```python
from build123d import *

# Parameters (mm, degrees)
PAD006_DEPTH    = 40
SKETCH009_W     = 14
SKETCH009_H     = 39
POCKET002_DEPTH = 5
SKETCH010_R     = 8.1
POCKET003_DEPTH = 5
FILLET001_R     = 3
FILLET002_R     = 2
FILLET003_R     = 4
CHAMFER_SIZE    = 2
CHAMFER001_SIZE = 2


with BuildPart() as part:
    # Sketch008 → Pad006 (new body, symmetric)
    with BuildSketch(Plane.YZ):
        Polygon((97.701339, 0), (115.394972, 0), (113.719903, 25.952241), (111.219903, 25.952241), (112.701339, 3), (97.701339, 3), align=None)
    extrude(amount=PAD006_DEPTH, both=True)

    # Sketch009 (on Face5 of Pad006) → Pocket002 (cut)
    with BuildSketch(Plane(origin=(0, 0, 3), x_dir=(0, -1, 0), z_dir=(0, 0, 1))):
        with Locations((-100.701339, 0)):
            Rectangle(SKETCH009_W, SKETCH009_H)
        with BuildLine():
            ThreePointArc((-103.101339, -36.625), (-101.401339, -38.325), (-99.701339, -36.625))
            Line((-99.701339, -36.625), (-99.701339, -33.225))
            ThreePointArc((-99.701339, -33.225), (-101.401339, -31.525), (-103.101339, -33.225))
            Line((-103.101339, -36.625), (-103.101339, -33.225))
        make_face()
        with BuildLine():
            ThreePointArc((-103.101339, 33.225), (-101.401339, 31.525), (-99.701339, 33.225))
            Line((-99.701339, 33.225), (-99.701339, 36.625))
            ThreePointArc((-99.701339, 36.625), (-101.401339, 38.325), (-103.101339, 36.625))
            Line((-103.101339, 33.225), (-103.101339, 36.625))
        make_face()
    extrude(amount=-POCKET002_DEPTH, mode=Mode.SUBTRACT)

    # Sketch010 (on Face3 of Pocket002) → Pocket003 (cut)
    with BuildSketch(Plane(origin=(0, 114.916235, 7.417187), x_dir=(0, -0.06441, 0.997924), z_dir=(0, 0.997924, 0.06441))):
        with Locations((12, -13)):
            Circle(SKETCH010_R)
        with Locations((12, 13)):
            Circle(SKETCH010_R)
    extrude(amount=-POCKET003_DEPTH, mode=Mode.SUBTRACT)

    # Fillet001
    fillet001_edges = [part.edges().sort_by_distance(p)[0] for p in [
        (-19.5, 97.701339, 1.5),
        (-40, 97.701339, 1.5),
        (19.5, 107.701339, 1.5),
        (19.5, 97.701339, 1.5),
        (40, 97.701339, 1.5),
        (-19.5, 107.701339, 1.5),
    ]]
    fillet(fillet001_edges, radius=FILLET001_R)

    # Fillet002
    fillet002_edges = [part.edges().sort_by_distance(p)[0] for p in [
        (-17.618693, 112.469704, 25.952241),
        (-8.381307, 112.469704, 25.952241),
        (8.381307, 112.469704, 25.952241),
        (17.618693, 112.469704, 25.952241),
    ]]
    fillet(fillet002_edges, radius=FILLET002_R)

    # Fillet003
    fillet003_edges = [part.edges().sort_by_distance(p)[0] for p in [
        (40, 112.469903, 25.952241),
    ]]
    fillet(fillet003_edges, radius=FILLET003_R)

    # Chamfer
    chamfer_edges = [part.edges().sort_by_distance(p)[0] for p in [
        (0, 112.701339, 3),
    ]]
    chamfer(chamfer_edges, length=CHAMFER_SIZE)

    # Chamfer001
    chamfer001_edges = [part.edges().sort_by_distance(p)[0] for p in [
        (0, 115.394972, 0),
    ]]
    chamfer(chamfer001_edges, length=CHAMFER001_SIZE)


with BuildPart() as part_1:
    # Body005 placement: moved
    add(part.part.moved(Location((0, 0, 3))))


solid = part_1.part
```
Source: CAD feature listing. Evaluate the final solid. Frame: model axes, mm. A direction names the side the tool comes from. Round coordinates to 2 decimals unless told otherwise and drop trailing zeros. Loops run counter-clockwise (first coordinate to the right, second up) from the corner with the lowest first, then second, coordinate; pieces in that order, holes last.
(1) Material intervals for probe 1 along Z at (x, y) = (-20.5, 99.5); probe 2 along Y at (x, z) = (13.5, 5); probe 3 along Y at (x, z) = (-8.5, 15.25), sorted ascending.
From the geometry:
probe 1: z = 3 to 6
probe 2: y = 107.7 to 115.27
probe 3: y = 112.1 to 114.6
(2) Section query B-B (y = 109.5). Output: boundary loops of the cut face in (x, z), and give its area (3 significant figures).
From the geometry:
outline: (-40, 3) - (40, 3) - (40, 6) - (-40, 6) - close
area: 240 mm2
(3) Section query C-C (z = 23.25). Give the number of separate pieces and of enclosed holes in the cut face, and give its area (3 significant figures).
From the geometry:
separate pieces: 3
enclosed holes: 0
area: 120 mm2
(4) Pull-direction query (X, two-part tool) for faces 1 (the flat face through (0.56, 114.676, 14.145)), 2 (the flat face through (-19.5, 103, 5)), 3 (the flat face through (-40, 113, 11)), 4 (the cylindrical face through (-12.767, 113.437, 14.233)); classes: +X half, -X half, draft (parallel to the pull), parting line (faces both ways), or undercut.
From the geometry:
face 1: draft
face 2: undercut
face 3: -X half
face 4: undercut
(5) Contact query for flat-ended pins moving along their axis: pin 1 Ø4 at (x, y) = (11.5, 104) entering from +Z; pin 2 Ø3.5 at (x, z) = (2, 5) entering from -Y; pin 3 Ø12 at (x, z) = (9, 18.5) entering from +Y. Output: stop coordinate, or through.
From the geometry:
pin 1: passes through
pin 2: stops at y = 107.7
pin 3: stops at y = 114.78
(6) Section query D-D (x = -12). Output: boundary loops of the cut face in (y, z), and give its area (3 significant figures).
From the geometry:
outline: (107.7, 3) - (113.39, 3) - (115.27, 5) - (114.66, 14.37) - (112.17, 14.21) - (112.57, 8) - (110.7, 6) - (107.7, 6) - close
area: 43.5 mm2
(7) Section query A-A (x = 30). Output: boundary loops of the cut face in (y, z).
From the geometry:
outline: (97.7, 3) - (113.39, 3) - (115.27, 5) - (113.72, 28.95) - (111.22, 28.95) - (112.57, 8) - (110.7, 6) - (97.7, 6) - close
(8) Access query for faces 5 (the cylindrical face through (20.36, 98.6, 4.48)), 6 (the flat face through (35, 103.101, 5)), 7 (the flat face through (0.56, 111.62, 6.98)), 8 (the flat face through (30, 97.701, 5)), 9 (the flat face through (29, 112, 28.952)). Directions: +Z, -Z, +X, -X, +Y, -Y. A direction counts if a zero-diameter tool reaches every point of the face in a straight line with its end or side. Return the directions, or none.
From the geometry:
face 5: +Z, -Z, -Y
face 6: +Z, -Z
face 7: +X, -X, -Y
face 8: +Z, -Z, +X, -X, -Y
face 9: +Z, +X, -X, +Y, -Y
